Could you check a few things on this model? Use its own coordinates, in mm. Coordinates: 2 decimals unless noted, no trailing zeros. Order: outer loops, then holes, each group sorted by start corner. A loop starts at its lowest first (then second) coordinate and runs counter-clockwise, first axis right, second up. Notation, with made-up numbers: M 67,55 L 116,55 A18 cw 116,67 Z; hole C 69.25,-20.5 d3. An arc over 180 degrees is marked long. Write item = value, one per line. Start each with the question number.
from build123d import *

# Parameters (mm, degrees)
HOLDER_OUTLINE_W                    = 25.3
HOLDER_OUTLINE_H                    = 62.6
F_2XAAA_HOLDER_25_3X62_6X15_5_DEPTH = 15.5
LONG_EDGE_FILLETS_R3_R              = 3
SLIDE_SWITCH_LEVER_SKETCH_W         = 3
SLIDE_SWITCH_LEVER_SKETCH_H         = 3
SLIDE_SWITCH_LEVER_3X3X1_3_DEPTH    = 1.3


with BuildPart() as part:
    # Holder Outline → 2xAAA Holder 25.3x62.6x15.5 (new body)
    with BuildSketch(Plane(origin=(0, 0, 0), x_dir=(1, 0, 0), z_dir=(0, 1, 0))):
        Rectangle(HOLDER_OUTLINE_W, HOLDER_OUTLINE_H)
    extrude(amount=F_2XAAA_HOLDER_25_3X62_6X15_5_DEPTH)

    # Long Edge Fillets R3
    long_edge_fillets_r3_edges = [part.edges().sort_by_distance(p)[0] for p in [
        (12.65, 15.5, 0),
        (-12.65, 15.5, 0),
        (12.65, 0, 0),
        (-12.65, 0, 0),
    ]]
    fillet(long_edge_fillets_r3_edges, radius=LONG_EDGE_FILLETS_R3_R)

    # Slide Switch Lever Sketch → Slide Switch Lever 3x3x1.3 (add)
    with BuildSketch(Plane(origin=(0, 0, 0), x_dir=(1, 0, 0), z_dir=(0, 1, 0))):
        with Locations((0, 25.3)):
            Rectangle(SLIDE_SWITCH_LEVER_SKETCH_W, SLIDE_SWITCH_LEVER_SKETCH_H)
    extrude(amount=-SLIDE_SWITCH_LEVER_3X3X1_3_DEPTH)


solid = part.part
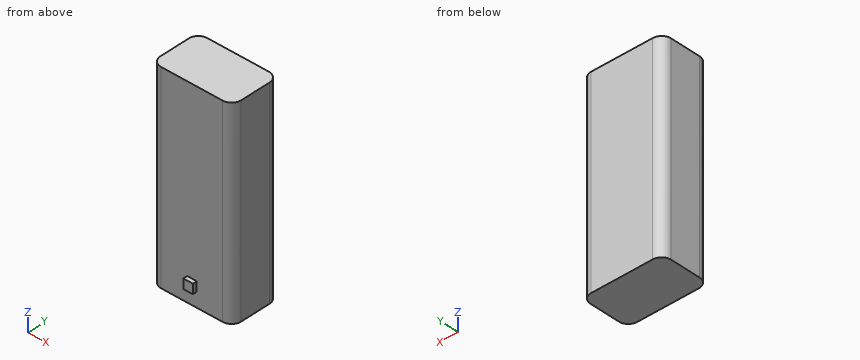
(1) Please list where these lines run through material, in increasing order: probe 1 along Y at (x, z) = (-9.75, -9); probe 2 along X at (y, z) = (1.5, 8); probe 3 along X at (y, z) = (13, -29). Write a range as from..to.
(2) Imagine slicing it at A-A on x = 0.5. List the corners of the cut face in (y, z) for me, plus the area to 3 significant figures.
(3) Imagine slicing it at C-C on y = 14. List the corners of the cut face in (x, z) for me.
(4) Imagine slicing it at D-D on x = -6.75. List the corners of the cut face in (y, z) for me.
(5) Will this pin go through, and if not, where does the flat tip stop? P1, Ø1.5, axis at x = 4.5, z = 20.5, coming from the -Y side.
(6) Imagine slicing it at B-B on z = 14. List the corners of the cut face in (x, y) for me, plus the area to 3 significant figures.
Response:
q1.probe_1 = 0..15.5
q1.probe_2 = -12.25..12.25
q1.probe_3 = -12.61..12.61
q2.outline = M -1.3,-26.8 L 0,-26.8 L 0,-31.3 L 15.5,-31.3 L 15.5,31.3 L 0,31.3 L 0,-23.8 L -1.3,-23.8 Z
q2.area = 974 mm2
q3.outline = M -12.25,-31.3 L 12.25,-31.3 L 12.25,31.3 L -12.25,31.3 Z
q4.outline = M 0,-31.3 L 15.5,-31.3 L 15.5,31.3 L 0,31.3 Z
q5.P1 = 0
q6.outline = M -12.65,3 A3 ccw -9.65,0 L 9.65,0 A3 ccw 12.65,3 L 12.65,12.5 A3 ccw 9.65,15.5 L -9.65,15.5 A3 ccw -12.65,12.5 Z
q6.area = 384 mm2
